The listing builds one solid part. Answer for the finished solid, in the listing's coordinates (mm). A direction names the side the tool comes from. Coordinates: 2 decimals unless noted, no trailing zeros. Loops run counter-clockwise (first coordinate to the right, second up) from the corner with the lowest first, then second, coordinate; pieces in that order, holes last. Notation, with made-up numbers: (-30, 32) - (8, 32) arc R24 ccw to (8, 71) - close; hole circle Ø1 at (39, 3.5). An arc over 180 degrees is marked (long way). Use one line per item in the form item = value. Start each with the question number.
```python
from build123d import *

# Parameters (mm, degrees)
F0_W     = 3.175
F0_H     = 19.05
F1_DEPTH = 20.955
F3_DEPTH = 45.72
F4_R     = 0.5
F5_DEPTH = 25.4


with BuildPart() as f1:
    # F0 (on Top) → F1 (new body)
    with BuildSketch(Plane.XY):
        Polygon((22.225, 48.458836), (-22.225, 48.458836), (-22.225, 10.358836), (-17.78, 10.358836), (17.78, 10.358836), (22.225, 10.358836), align=None)
        Polygon((17.78, 10.358836), (-17.78, 10.358836), (-17.78, -8.691164), (-14.605, -8.691164), (14.605, -8.691164), (17.78, -8.691164), align=None)
        with Locations((-16.1925, -18.216164)):
            Rectangle(F0_W, F0_H)
        with Locations((16.1925, -18.216164)):
            Rectangle(F0_W, F0_H)
    extrude(amount=F1_DEPTH)

    # F2 (on face) → F3 (cut)
    with BuildSketch(Plane(origin=(-17.78, 0, 0), x_dir=(0, -1, 0), z_dir=(-1, 0, 0))):
        Polygon((19.486164, 13.6525), (27.741164, 13.6525), (27.741164, 20.955), (3.611164, 20.955), (3.611164, 16.8148), (19.486164, 16.8148), align=None)
        Polygon((27.741164, 0), (27.741164, 7.3025), (19.486164, 7.3025), (19.486164, 4.1148), (3.611164, 4.1148), (3.611164, 0), align=None)
    extrude(amount=-F3_DEPTH, mode=Mode.SUBTRACT)

    # F4 (on face) → F5 (join)
    with BuildSketch(Plane(origin=(-22.225, 0, 0), x_dir=(0, -1, 0), z_dir=(-1, 0, 0))):
        with Locations((-32.797098, 9.996843)):
            Circle(F4_R)
    extrude(amount=F5_DEPTH)

    # F6: F1 across plane


with BuildPart() as f1_1:
    add(f1.part)
    add(f1.part.mirror(Plane.YZ))


solid = f1_1.part
```
(1) A cutting plane is placed at B-B (z = 3). Determine the outline of the cut face in (x, y) (3 decimals), then the cut area to 3 significant figures.
(2) Each of these flat-tipped pins is pushed along its axis until it touches: pin 1 Ø1 at (x, y) = (16.5, -25) entering from +Z; pin 2 Ø1.6 at (x, y) = (-16.5, -22) entering from -Z; pin 3 Ø6 at (y, z) = (21, 5.5) entering from -X (3 decimals). Where does it stop, or does it pass through?
(3) A cutting plane is placed at D-D (z = 15.5). Determine the outline of the cut face in (x, y) (3 decimals), then the cut area to 3 significant figures.
(4) A cutting plane is placed at C-C (x = 0.5). Determine the outline of the cut face in (y, z) (3 decimals).
(5) For faces 1 (the face through (-17.78, -4, 10)), 2 (the face through (16, -24, 7.302)), 3 (the face through (20, 10.359, 10)), 4 (the face through (0, -8.691, 10)), 5 (the face through (16, -19.486, 15)), determine the directions among +Z, -Z, +X, -X, +Y, -Y from which every point of the face is accessible in a straight line to the end or side of a thin tool.
(6) Find the intervals of material crossed by probe 1 along X at (y, z) = (21.5, 18.75) (3 decimals); probe 2 along X at (y, z) = (8.5, 8.25); probe 3 along Y at (x, z) = (-9, 12.5), in increasing order. Write a range as from..to.
(7) A cutting plane is placed at A-A (y = -21.5). Determine the outline of the cut face in (x, z) (1 decimal).
Evaluation:
q1.outline = (-22.225, 10.359) - (-17.78, 10.359) - (-17.78, -3.611) - (17.78, -3.611) - (17.78, 10.359) - (22.225, 10.359) - (22.225, 48.459) - (-22.225, 48.459) - close
q1.area = 2,190 mm^2
q2.pin_1 = 13.65
q2.pin_2 = 7.3
q2.pin_3 = -22.225
q3.outline = (-22.225, 10.359) - (-17.78, 10.359) - (-17.78, -19.486) - (-14.605, -19.486) - (-14.605, -8.691) - (14.605, -8.691) - (14.605, -19.486) - (17.78, -19.486) - (17.78, 10.359) - (22.225, 10.359) - (22.225, 48.459) - (-22.225, 48.459) - close
q3.area = 2,440 mm^2
q4.outline = (-8.691, 4.115) - (-3.611, 4.115) - (-3.611, 0) - (48.459, 0) - (48.459, 20.955) - (-3.611, 20.955) - (-3.611, 16.815) - (-8.691, 16.815) - close
q5.face_1 = +Z, -Z, -X, -Y
q5.face_2 = -Z, +X, -X, -Y
q5.face_3 = +Z, -Z, +X, -Y
q5.face_4 = +Z, -Z, -Y
q5.face_5 = +Z, +X, -X, -Y
q6.probe_1 = -22.225..22.225
q6.probe_2 = -17.78..17.78
q6.probe_3 = -8.69..48.46
q7.outline = (-17.8, 7.3) - (-14.6, 7.3) - (-14.6, 13.7) - (-17.8, 13.7) - close; (14.6, 7.3) - (17.8, 7.3) - (17.8, 13.7) - (14.6, 13.7) - close
